For this review, take the finished solid that the model builds, in its own axes (mm). A direction names the side the tool comes from. Round coordinates to 2 decimals unless told otherwise and drop trailing zeros. Loops run counter-clockwise (first coordinate to the right, second up) from the corner with the lowest first, then second, coordinate; pieces in that order, holes last.
```python
from build123d import *

# Parameters (mm, degrees)
SKETCH2_R          = 4
CUT_EXTRUDE1_DEPTH = 18.875437058
SKETCH3_W          = 3.15
SKETCH3_H          = 4
CUT_EXTRUDE2_DEPTH = 21.417302711
FILLET1_R          = 0.5
FILLET2_R          = 0.25
CHAMFER1_SIZE      = 0.75


with BuildPart() as part:
    # Sketch1 → Revolve1 (revolve)
    with BuildSketch(Plane.XY):
        Polygon((0, 0), (-6.875, 0), (-6.875, 4), (-5.15, 4), (-5.15, 15), (0, 15), align=None)
    revolve(axis=Axis((0, 15, 0), (0, -1, 0)))

    # Sketch2 → Cut-Extrude1 (cut, through all)
    with BuildSketch(Plane(origin=(0, 15, 0), x_dir=(1, 0, 0), z_dir=(0, 1, 0))):
        with Locations(Location((0, 0, 0), (0, 0, 180))):
            Circle(SKETCH2_R)
    extrude(amount=-CUT_EXTRUDE1_DEPTH, mode=Mode.SUBTRACT)

    # Sketch3 → Cut-Extrude2 (cut, through all)
    with BuildSketch(Plane(origin=(5.15, 0, 0), x_dir=(0, 0, -1), z_dir=(1, 0, 0))):
        with Locations((-3.575, 13)):
            Rectangle(SKETCH3_W, SKETCH3_H)
        with Locations((3.575, 13)):
            Rectangle(SKETCH3_W, SKETCH3_H)
    extrude(amount=-CUT_EXTRUDE2_DEPTH, mode=Mode.SUBTRACT)

    # Fillet1
    fillet1_edges = [part.edges().sort_by_distance(p)[0] for p in [
        (5.15, 4, 0),
    ]]
    fillet(fillet1_edges, radius=FILLET1_R)

    # Fillet2
    fillet2_edges = [part.edges().sort_by_distance(p)[0] for p in [
        (6.875, 4, 0),
        (6.875, 0, 0),
    ]]
    fillet(fillet2_edges, radius=FILLET2_R)

    # Chamfer1
    chamfer1_edges = [part.edges().sort_by_distance(p)[0] for p in [
        (4, 0, 0),
    ]]
    chamfer(chamfer1_edges, length=CHAMFER1_SIZE)


solid = part.part
```
(1) For L1, parallel to X at y = 9.5, z = 0; L2, parallel to X at y = 2, z = 1.25, list the stretches that pass through material, from the lowest coordinate up.
(2) Add section C-C (z = 0). Give the boundary of the cut face in (x, y) (3 decimals), plus the area to 3 significant figures.
(3) Add section A-A (x = 0). Give the boundary of the cut face in (y, z) (3 decimals).
(4) For faces 1 (the flat face through (-5, 4, -3)), 2 (the flat face through (-4, 13, -2)), 3 (the cylindrical face through (1.49, 2.02, 6.71)), 4 (the flat face through (-4, 13, 2)), 5 (the flat face through (-4.5, 15, 0)), list the 3-axis set-ups (+Z, -Z, +X, -X, +Y, -Y) from which the entire face can be reached by the end or side of a thin tool; tool diameter is ignored.
(5) The part is to be moulded in two halves that separate along X. For faces 6 (the cylindrical face through (-3.695, 6.391, -1.532)), 7 (the cylindrical face through (-4.91, 8.66, -1.55)), 8 (the flat face through (0.1, 11, -4.3)), say which applies: pulls with the +X half, pulls with the -X half, needs draft (parallel to the pull), parting line crosses it, or undercut.
(6) Add section D-D (y = 7.5). Give the boundary of the cut face in (x, z), plus the area to 3 significant figures.
(7) Insertion check: pin 1 Ø2 at (x, z) = (-1, -2) entering from -Y; pin 2 Ø5 at (x, y) = (-1, 2.5) entering from -Z (3 decimals); pin 3 Ø1.5 at (x, y) = (3.5, 13.5) entering from +Z; pin 4 Ø0.9 at (x, z) = (-2.5, 3.5) entering from +Y. Each pin has a flat end and moves straight along its axis. Give the tip position at first contact, or say it passes through.
(8) Add section B-B (y = 12). Give the boundary of the cut face in (x, z).
Outcome:
1. L1: x = -5.15 to -4, 4 to 5.15
1. L2: x = -6.76 to -3.8, 3.8 to 6.76
2. outline: (-6.875, 0.25) arc R0.25 ccw to (-6.625, 0) - (-4.75, 0) - (-4, 0.75) - (-4, 15) - (-5.15, 15) - (-5.15, 4.5) arc R0.5 cw to (-5.65, 4) - (-6.625, 4) arc R0.25 ccw to (-6.875, 3.75) - close; (4, 0.75) - (4.75, 0) - (6.625, 0) arc R0.25 ccw to (6.875, 0.25) - (6.875, 3.75) arc R0.25 ccw to (6.625, 4) - (5.65, 4) arc R0.5 cw to (5.15, 4.5) - (5.15, 15) - (4, 15) - close
2. area: 47.8 mm2
3. outline: (0, -6.625) arc R0.25 ccw to (0.25, -6.875) - (3.75, -6.875) arc R0.25 ccw to (4, -6.625) - (4, -5.65) arc R0.5 cw to (4.5, -5.15) - (11, -5.15) - (11, -4) - (0.75, -4) - (0, -4.75) - close; (0, 4.75) - (0.75, 4) - (11, 4) - (11, 5.15) - (4.5, 5.15) arc R0.5 cw to (4, 5.65) - (4, 6.625) arc R0.25 ccw to (3.75, 6.875) - (0.25, 6.875) arc R0.25 ccw to (0, 6.625) - close
4. face 1: +Y
4. face 2: -Z, +X, -X, +Y
4. face 3: +Y, -Y
4. face 4: +Z, +X, -X, +Y
4. face 5: +Z, -Z, +X, -X, +Y
5. face 6: undercut
5. face 7: parting line crosses it
5. face 8: needs draft
6. outline: circle Ø10.3 at (0, 0); hole circle Ø8 at (0, 0)
6. area: 33.1 mm2
7. pin 1: passes through
7. pin 2: stops at z = -6.875
7. pin 3: stops at z = 2
7. pin 4: stops at y = 11
8. outline: (-4.75, -2) - (-3.46, -2) arc R4 cw to (-3.46, 2) - (-4.75, 2) arc R5.15 ccw to start; (3.46, -2) - (4.75, -2) arc R5.15 ccw to (4.75, 2) - (3.46, 2) arc R4 cw to start
